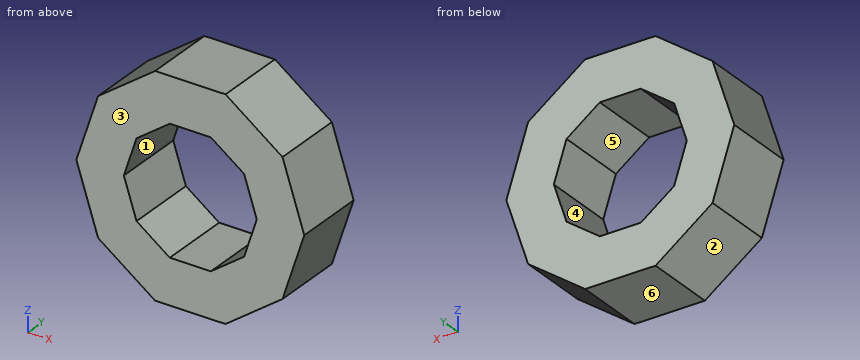
from build123d import *

# Parameters (mm, degrees)
F1_DEPTH = 25.4


with BuildPart() as f1:
    # F0 (on Front) → F1 (new body)
    with BuildSketch(Plane.XZ):
        Polygon((12.37944, 38.1), (0, 38.1), (-12.37944, 38.1), (-32.409796, 23.547095), (-40.060711, 0), (-32.409796, -23.547095), (-12.37944, -38.1), (12.37944, -38.1), (32.409796, -23.547095), (40.060711, 0), (32.409796, 23.547095), align=None)
        Polygon((-7.22134, 22.225), (0, 22.225), (7.22134, 22.225), (18.905714, 13.735805), (23.368748, 0), (18.905714, -13.735805), (7.22134, -22.225), (-7.22134, -22.225), (-18.905714, -13.735805), (-23.368748, 0), (-18.905714, 13.735805), align=None, mode=Mode.SUBTRACT)
    extrude(amount=F1_DEPTH)


solid = f1.part
Design review of the part built by this model. Coordinates are the model's own, in mm. Face numbers are marked on the shaded views. A direction names the side the tool comes from. Coordinates: 2 decimals unless noted, no trailing zeros. Write each loop counter-clockwise with the first axis right and the second up, starting at its lowest first coordinate (ties: lowest second). Pieces come first, ordered by that corner, then holes. Notation, with made-up numbers: (49.25, -26.5) - (99.25, -26.5) arc R19 cw to (99.25, -2.5) - close; hole circle Ø1 at (-37, 41). An arc over 180 degrees is marked (long way). One line per item, written item: value.
1) Add section B-B (z = 17). State the section outline as (x, y) points.
Answer sheet:
outline: (-34.54, -25.4) - (-14.41, -25.4) - (-14.41, 0) - (-34.54, 0) - close; (14.41, -25.4) - (34.54, -25.4) - (34.54, 0) - (14.41, 0) - close
2) For the marked faces 5 and 6, list the 3-axis set-ups (+Z, -Z, +X, -X, +Y, -Y) from which the entire face can be reached by the end or side of a thin tool; tool diameter is ignored.
Answer sheet:
face 5: +Y, -Y
face 6: -Z, +X, -X, +Y, -Y
3) To check wall thickness, follow probe 1 along Z at (x, y) = (-4, -12.5) (3 decimals); probe 2 along Z at (x, y) = (9.5, -6.5); probe 3 along X at (y, z) = (-15.5, -18.5). State the ranges of each line that lie inside material, in increasing order.
Answer sheet:
probe 1: z = -38.1 to -22.225, 22.225 to 38.1
probe 2: z = -38.1 to -20.57, 20.57 to 38.1
probe 3: x = -34.05 to -12.35, 12.35 to 34.05
4) Add section A-A (y = -19). State the section outline as (x, z) points (3 decimals).
Answer sheet:
outline: (-40.061, 0) - (-32.41, -23.547) - (-12.379, -38.1) - (12.379, -38.1) - (32.41, -23.547) - (40.061, 0) - (32.41, 23.547) - (12.379, 38.1) - (-12.379, 38.1) - (-32.41, 23.547) - close; hole (-23.369, 0) - (-18.906, -13.736) - (-7.221, -22.225) - (7.221, -22.225) - (18.906, -13.736) - (23.369, 0) - (18.906, 13.736) - (7.221, 22.225) - (-7.221, 22.225) - (-18.906, 13.736) - close
5) Add section C-C (x = -8.5). State the section outline as (y, z) points, plus the area to 3 significant figures.
Answer sheet:
outline: (-25.4, -38.1) - (0, -38.1) - (0, -21.3) - (-25.4, -21.3) - close; (-25.4, 21.3) - (0, 21.3) - (0, 38.1) - (-25.4, 38.1) - close
area: 854 mm2
6) Mouldability with a two-part tool opening along X and no side actions: class the marked faces 1, 2, 3 and 4 as +X half, -X half, draft (parallel to the pull), parting line (faces both ways), or undercut.
Answer sheet:
face 1: undercut
face 2: -X half
face 3: draft
face 4: undercut
7) Add section D-D (x = 26). State the section outline as (y, z) points, plus the area to 3 significant figures.
Answer sheet:
outline: (-25.4, -28.2) - (0, -28.2) - (0, 28.2) - (-25.4, 28.2) - close
area: 1,430 mm2
8) Insertion check: pin 1 (5 mm diameter, centred on y = -4, z = -28.5, fed in from -X); pin 2 (10 mm diameter, centred on x = 25, y = -6, fed in from +Z). Each pin has a flat end and moves straight along its axis. Give the tip position at first contact, or say it passes through.
Answer sheet:
pin 1: stops at x = -29.03
pin 2: stops at z = 32.56
